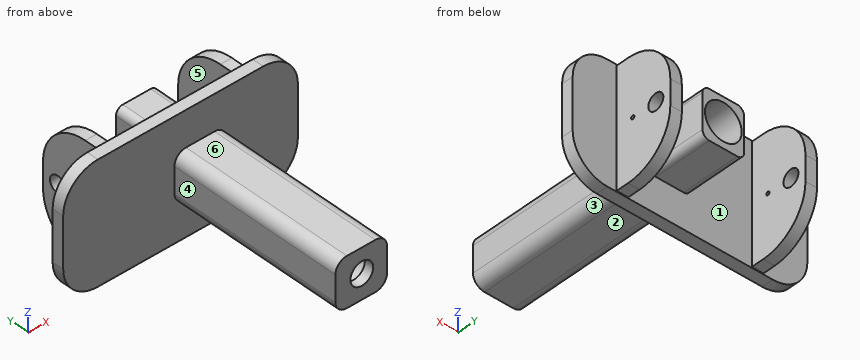
```python
from build123d import *

# Parameters (mm, degrees)
SKETCH2_W           = 101.6
SKETCH2_H           = 101.6
BOSS_EXTRUDE2_DEPTH = 5
SKETCH3_W           = 5
SKETCH3_H           = 50.8
BOSS_EXTRUDE3_DEPTH = 25.4
SKETCH4_W           = 5
SKETCH4_H           = 50.8
BOSS_EXTRUDE4_DEPTH = 25.4
SKETCH8_R           = 3.556
CUT_EXTRUDE1_DEPTH  = 135.392047756
CUT_EXTRUDE2_REACH  = 136.392
SKETCH9_R           = 0.762
SKETCH11_R          = 7.9502
CUT_EXTRUDE3_DEPTH  = 146.911891222
CUT_EXTRUDE5_REACH  = 136.392
SKETCH18_R          = 0.762
SKETCH19_W          = 22.350467385
SKETCH19_H          = 21.198381437
BOSS_EXTRUDE5_DEPTH = 76.2
SKETCH22_R          = 7.94
CUT_EXTRUDE7_DEPTH  = 72.2
SKETCH23_R          = 4.95
CUT_EXTRUDE8_DEPTH  = 179.909697893
SKETCH24_W          = 101.6
SKETCH24_H          = 25
CUT_EXTRUDE9_DEPTH  = 166.041085794
SKETCH25_W          = 101.6
SKETCH25_H          = 25
CUT_EXTRUDE10_DEPTH = 166.041085794
FILLET1_R           = 20
FILLET2_R           = 20
FILLET3_R           = 20
FILLET4_R           = 20
FILLET5_R           = 15
FILLET6_R           = 15
FILLET7_R           = 15
FILLET8_R           = 15
FILLET9_R           = 5
FILLET10_R          = 5
FILLET11_R          = 5
FILLET12_R          = 5
SKETCH35_W          = 18
SKETCH35_H          = 21
BOSS_EXTRUDE7_DEPTH = 25.4
CUT_EXTRUDE12_REACH = 167.993
SKETCH36_R          = 7.95
FILLET18_R          = 3
FILLET19_R          = 3
FILLET20_R          = 3
FILLET21_R          = 3


with BuildPart() as part:
    # Sketch2 → Boss-Extrude2 (new body)
    with BuildSketch(Plane(origin=(0, 0, 0), x_dir=(1, 0, 0), z_dir=(0, 1, 0))):
        with Locations((50.8, -50.8)):
            Rectangle(SKETCH2_W, SKETCH2_H)
    extrude(amount=BOSS_EXTRUDE2_DEPTH)

    # Sketch3 → Boss-Extrude3 (add)
    with BuildSketch(Plane(origin=(0, 5, 0), x_dir=(1, 0, 0), z_dir=(0, 1, 0))):
        with Locations((21.55, -50.8)):
            Rectangle(SKETCH3_W, SKETCH3_H)
    extrude(amount=BOSS_EXTRUDE3_DEPTH)

    # Sketch4 → Boss-Extrude4 (add)
    with BuildSketch(Plane(origin=(0, 5, 0), x_dir=(1, 0, 0), z_dir=(0, 1, 0))):
        with Locations((80.05, -50.8)):
            Rectangle(SKETCH4_W, SKETCH4_H)
    extrude(amount=BOSS_EXTRUDE4_DEPTH)

    # Sketch8 → Cut-Extrude1 (cut, through all)
    with BuildSketch(Plane.ZY.offset(-19.05)):
        with Locations((50.8, 23.542)):
            Circle(SKETCH8_R)
    extrude(amount=-CUT_EXTRUDE1_DEPTH, mode=Mode.SUBTRACT)

    # Sketch9 → Cut-Extrude2 (cut, up to next)
    with BuildSketch(Plane(origin=(82.55, 0, 0), x_dir=(0, 0, -1), z_dir=(1, 0, 0)), mode=Mode.PRIVATE) as cut_extrude2_sk1:
        with Locations((-50.8, 12.62)):
            Circle(SKETCH9_R)
    cut_extrude2_tool1 = extrude(cut_extrude2_sk1.sketch, amount=-CUT_EXTRUDE2_REACH, mode=Mode.PRIVATE) & part.part
    add(cut_extrude2_tool1.solids().sort_by_distance((82.55, 12.62, 50.8))[0], mode=Mode.SUBTRACT)

    # Sketch11 → Cut-Extrude3 (cut, through all)
    with BuildSketch(Plane(origin=(0, 5, 0), x_dir=(1, 0, 0), z_dir=(0, 1, 0))):
        with Locations(Location((59.61, -50.8, 0), (0, 0, 270))):
            Circle(SKETCH11_R)
    extrude(amount=-CUT_EXTRUDE3_DEPTH, mode=Mode.SUBTRACT)

    # Sketch18 → Cut-Extrude5 (cut, up to next)
    with BuildSketch(Plane.ZY.offset(-19.05), mode=Mode.PRIVATE) as cut_extrude5_sk1:
        with Locations(Location((50.8, 12.62, 0), (0, 0, 180))):
            Circle(SKETCH18_R)
    cut_extrude5_tool1 = extrude(cut_extrude5_sk1.sketch, amount=-CUT_EXTRUDE5_REACH, mode=Mode.PRIVATE) & part.part
    add(cut_extrude5_tool1.solids().sort_by_distance((19.05, 12.62, 50.8))[0], mode=Mode.SUBTRACT)

    # Sketch19 → Boss-Extrude5 (add)
    with BuildSketch(Plane.XZ):
        with Locations((59.324658632, 50.761526183)):
            Rectangle(SKETCH19_W, SKETCH19_H)
    extrude(amount=BOSS_EXTRUDE5_DEPTH)

    # Sketch22 → Cut-Extrude7 (cut)
    with BuildSketch(Plane(origin=(0, 0, 0), x_dir=(1, 0, 0), z_dir=(0, 1, 0))):
        with Locations(Location((59.61, -50.8, 0), (0, 0, 270))):
            Circle(SKETCH22_R)
    extrude(amount=-CUT_EXTRUDE7_DEPTH, mode=Mode.SUBTRACT)

    # Sketch23 → Cut-Extrude8 (cut, through all)
    with BuildSketch(Plane.XZ.offset(76.2)):
        with Locations(Location((59.61, 50.8, 0), (0, 0, 270))):
            Circle(SKETCH23_R)
    extrude(amount=-CUT_EXTRUDE8_DEPTH, mode=Mode.SUBTRACT)

    # Sketch24 → Cut-Extrude9 (cut, through all)
    with BuildSketch(Plane(origin=(0, 5, 0), x_dir=(1, 0, 0), z_dir=(0, 1, 0))):
        with Locations((50.8, -12.5)):
            Rectangle(SKETCH24_W, SKETCH24_H)
    extrude(amount=-CUT_EXTRUDE9_DEPTH, mode=Mode.SUBTRACT)

    # Sketch25 → Cut-Extrude10 (cut, through all)
    with BuildSketch(Plane(origin=(0, 5, 0), x_dir=(1, 0, 0), z_dir=(0, 1, 0))):
        with Locations((50.8, -89.1)):
            Rectangle(SKETCH25_W, SKETCH25_H)
    extrude(amount=-CUT_EXTRUDE10_DEPTH, mode=Mode.SUBTRACT)

    # Fillet1
    fillet1_edges = [part.edges().sort_by_distance(p)[0] for p in [
        (21.55, 30.4, 76.2),
    ]]
    fillet(fillet1_edges, radius=FILLET1_R)

    # Fillet2
    fillet2_edges = [part.edges().sort_by_distance(p)[0] for p in [
        (21.55, 30.4, 25.4),
    ]]
    fillet(fillet2_edges, radius=FILLET2_R)

    # Fillet3
    fillet3_edges = [part.edges().sort_by_distance(p)[0] for p in [
        (80.05, 30.4, 25.4),
    ]]
    fillet(fillet3_edges, radius=FILLET3_R)

    # Fillet4
    fillet4_edges = [part.edges().sort_by_distance(p)[0] for p in [
        (80.05, 30.4, 76.2),
    ]]
    fillet(fillet4_edges, radius=FILLET4_R)

    # Fillet5
    fillet5_edges = [part.edges().sort_by_distance(p)[0] for p in [
        (101.6, 2.5, 76.6),
    ]]
    fillet(fillet5_edges, radius=FILLET5_R)

    # Fillet6
    fillet6_edges = [part.edges().sort_by_distance(p)[0] for p in [
        (101.6, 2.5, 25),
    ]]
    fillet(fillet6_edges, radius=FILLET6_R)

    # Fillet7
    fillet7_edges = [part.edges().sort_by_distance(p)[0] for p in [
        (0, 2.5, 25),
    ]]
    fillet(fillet7_edges, radius=FILLET7_R)

    # Fillet8
    fillet8_edges = [part.edges().sort_by_distance(p)[0] for p in [
        (0, 2.5, 76.6),
    ]]
    fillet(fillet8_edges, radius=FILLET8_R)

    # Fillet9
    fillet9_edges = [part.edges().sort_by_distance(p)[0] for p in [
        (70.499892324, -38.1, 61.360716901),
    ]]
    fillet(fillet9_edges, radius=FILLET9_R)

    # Fillet10
    fillet10_edges = [part.edges().sort_by_distance(p)[0] for p in [
        (70.499892324, -38.1, 40.162335464),
    ]]
    fillet(fillet10_edges, radius=FILLET10_R)

    # Fillet11
    fillet11_edges = [part.edges().sort_by_distance(p)[0] for p in [
        (48.149424939, -38.1, 61.360716901),
    ]]
    fillet(fillet11_edges, radius=FILLET11_R)

    # Fillet12
    fillet12_edges = [part.edges().sort_by_distance(p)[0] for p in [
        (48.149424939, -38.1, 40.162335464),
    ]]
    fillet(fillet12_edges, radius=FILLET12_R)

    # Sketch35 → Boss-Extrude7 (add)
    with BuildSketch(Plane(origin=(0, 5, 0), x_dir=(1, 0, 0), z_dir=(0, 1, 0))):
        with Locations((59.61, -50.5)):
            Rectangle(SKETCH35_W, SKETCH35_H)
    extrude(amount=BOSS_EXTRUDE7_DEPTH)

    # Sketch36 → Cut-Extrude12 (cut, up to next)
    with BuildSketch(Plane(origin=(0, 30.4, 0), x_dir=(1, 0, 0), z_dir=(0, 1, 0)), mode=Mode.PRIVATE) as cut_extrude12_sk1:
        with Locations(Location((59.61, -50.8, 0), (0, 0, 270))):
            Circle(SKETCH36_R)
    cut_extrude12_tool1 = extrude(cut_extrude12_sk1.sketch, amount=-CUT_EXTRUDE12_REACH, mode=Mode.PRIVATE) & part.part
    add(cut_extrude12_tool1.solids().sort_by_distance((59.61, 30.4, 50.8))[0], mode=Mode.SUBTRACT)

    # Fillet18
    fillet18_edges = [part.edges().sort_by_distance(p)[0] for p in [
        (50.61, 17.7, 61),
    ]]
    fillet(fillet18_edges, radius=FILLET18_R)

    # Fillet19
    fillet19_edges = [part.edges().sort_by_distance(p)[0] for p in [
        (68.61, 17.7, 61),
    ]]
    fillet(fillet19_edges, radius=FILLET19_R)

    # Fillet20
    fillet20_edges = [part.edges().sort_by_distance(p)[0] for p in [
        (68.61, 17.7, 40),
    ]]
    fillet(fillet20_edges, radius=FILLET20_R)

    # Fillet21
    fillet21_edges = [part.edges().sort_by_distance(p)[0] for p in [
        (50.61, 17.7, 40),
    ]]
    fillet(fillet21_edges, radius=FILLET21_R)


solid = part.part
```
Build history of the part. All positions in model axes, mm. Face numbers are marked on the shaded views. A direction names the side the tool comes from. Round coordinates to 2 decimals unless told otherwise and drop trailing zeros. Loops run counter-clockwise (first coordinate to the right, second up) from the corner with the lowest first, then second, coordinate; pieces in that order, holes last.
Item 1: Drill centre lines: line 1 along Z through (x, y) = (59, -19); line 2 along X through (y, z) = (3.3, 50.8); line 3 along X through (y, z) = (23.75, 50.8). Where is each one in solid material? Low to high.
Item 2: Two-plate mould, pull along X, no slides. Class the marked faces 1, 2 and 3: released by +X, released by -X, zero draft, split by the parting line, or undercut.
Item 3: Saw through at C-C (z = 37). List the corners of the cut face in (x, y), then the cut area to 3 significant figures.
Item 4: Saw through at D-D (z = 30.5). List the corners of the cut face in (x, y).
Item 5: Saw through at A-A (y = -14). List the corners of the cut face in (x, z), then the cut area to 3 significant figures.
Item 6: Which spindle directions (+Z, -Z, +X, -X, +Y, -Y) get a long thin tool onto all of the face, cutting with end or side? Do the marked faces 4, 5 and 6. Say none if no direction does.
Item 7: Pin check, flat tips, straight feed: P1, Ø6, axis at x = 78, z = 63.5, coming from the +Y side; P2, Ø3.5, axis at x = 58.5, y = 20, coming from the +Z side; P3, Ø5, axis at y = 9, z = 43, coming from the -X side; P4, Ø9, axis at x = 59.61, z = 50.8, coming from the +Y side. Stop position of each tip, or through.
Worked answers:
1. line 1: z = 40.16 to 42.88, 58.72 to 61.36
1. line 2: x = 0 to 51.66, 67.56 to 101.6
1. line 3: x = 50.61 to 51.66, 67.56 to 68.61
2. face 1: undercut
2. face 2: zero draft
2. face 3: released by +X
3. outline: (0.3, 0) - (101.3, 0) - (101.3, 5) - (82.55, 5) - (82.55, 28.55) - (77.55, 28.55) - (77.55, 5) - (24.05, 5) - (24.05, 28.55) - (19.05, 28.55) - (19.05, 5) - (0.3, 5) - close
3. area: 740 mm2
4. outline: (3.39, 0) - (98.21, 0) - (98.21, 5) - (82.55, 5) - (82.55, 23.74) - (77.55, 23.74) - (77.55, 5) - (24.05, 5) - (24.05, 23.74) - (19.05, 23.74) - (19.05, 5) - (3.39, 5) - close
5. outline: (48.15, 45.16) arc R5 ccw to (53.15, 40.16) - (65.5, 40.16) arc R5 ccw to (70.5, 45.16) - (70.5, 56.36) arc R5 ccw to (65.5, 61.36) - (53.15, 61.36) arc R5 ccw to (48.15, 56.36) - close; hole circle Ø15.88 at (59.61, 50.8)
5. area: 254 mm2
6. face 4: +Z, -Z, -X, -Y
6. face 5: +Z, -Z, +Y
6. face 6: +Z, +X, -X, -Y
7. P1: stops at y = 29.93
7. P2: stops at z = 61
7. P3: stops at x = 19.05
7. P4: passes through
